The model under review builds one solid part; all positions refer to its coordinate system, in mm. A direction names the side the tool comes from. Round coordinates to 2 decimals unless told otherwise and drop trailing zeros. One line per item, written item: value. Start each with the question number.
1) Wall thickness on probe 1 along X at (y, z) = (240, 1.45); probe 2 along Y at (x, z) = (310, 1.5); probe 3 along Y at (x, z) = (160.5, 5): over which ranges is each line inside the solid? List them lowest first.
2) For P1, Ø9.5, axis at x = 160, y = 350, coming from the +Z side; P2, Ø8.5, axis at x = 308.5, y = 240, coming from the +Z side, all flat-tipped, find the tip position at first contact; note any pin that passes through.
3) Mouldability with a two-part tool opening along X and no side actions: class faces 3 (the face through (154.805, 10.229, 4.774)), 4 (the face through (158, 183, 0)) as +X half, -X half, draft (parallel to the pull), parting line (faces both ways), or undercut.
4) Tool access review of faces 1 (the face through (155.9, 346.8, 4.8)), 2 (the face through (158, 183, 6.5)): name each direction out of +Z, -Z, +X, -X, +Y, -Y from which nothing blocks a thin tool from reaching the whole face with its end or side.
from build123d import *

# Parameters (mm, degrees)
SKETCH_W        = 320
SKETCH_H        = 360
PAD_DEPTH       = 6.5
SKETCH001_R     = 5.2
POCKET_DEPTH    = 3.5
SKETCH002_R     = 3.2
POCKET001_DEPTH = 3


with BuildPart() as part:
    # Sketch → Pad (new body)
    with BuildSketch(Plane.XY):
        with Locations((160, 180)):
            Rectangle(SKETCH_W, SKETCH_H)
    extrude(amount=PAD_DEPTH)

    # Sketch001 (on Face6 of Pad) → Pocket (cut)
    with BuildSketch(Plane.XY.offset(6.5)):
        with Locations((160, 350)):
            Circle(SKETCH001_R)
        with Locations((310, 240)):
            Circle(SKETCH001_R)
        with Locations((310, 120)):
            Circle(SKETCH001_R)
        with Locations((160, 10)):
            Circle(SKETCH001_R)
        with Locations((10, 120)):
            Circle(SKETCH001_R)
        with Locations((10, 240)):
            Circle(SKETCH001_R)
    extrude(amount=-POCKET_DEPTH, mode=Mode.SUBTRACT)

    # Sketch002 (on Face17 of Pocket) → Pocket001 (cut)
    with BuildSketch(Plane.XY.offset(3)):
        with Locations((160, 350)):
            Circle(SKETCH002_R)
        with Locations((10, 240)):
            Circle(SKETCH002_R)
        with Locations((10, 120)):
            Circle(SKETCH002_R)
        with Locations((160, 10)):
            Circle(SKETCH002_R)
        with Locations((310, 120)):
            Circle(SKETCH002_R)
        with Locations((310, 240)):
            Circle(SKETCH002_R)
    extrude(amount=-POCKET001_DEPTH, mode=Mode.SUBTRACT)


solid = part.part
Checked values:
1. probe 1: x = 0 to 6.8, 13.2 to 306.8, 313.2 to 320
1. probe 2: y = 0 to 116.8, 123.2 to 236.8, 243.2 to 360
1. probe 3: y = 0 to 4.82, 15.18 to 344.82, 355.18 to 360
2. P1: stops at z = 3
2. P2: stops at z = 6.5
3. face 3: undercut
3. face 4: draft
4. face 1: +Z
4. face 2: +Z, +X, -X, +Y, -Y
